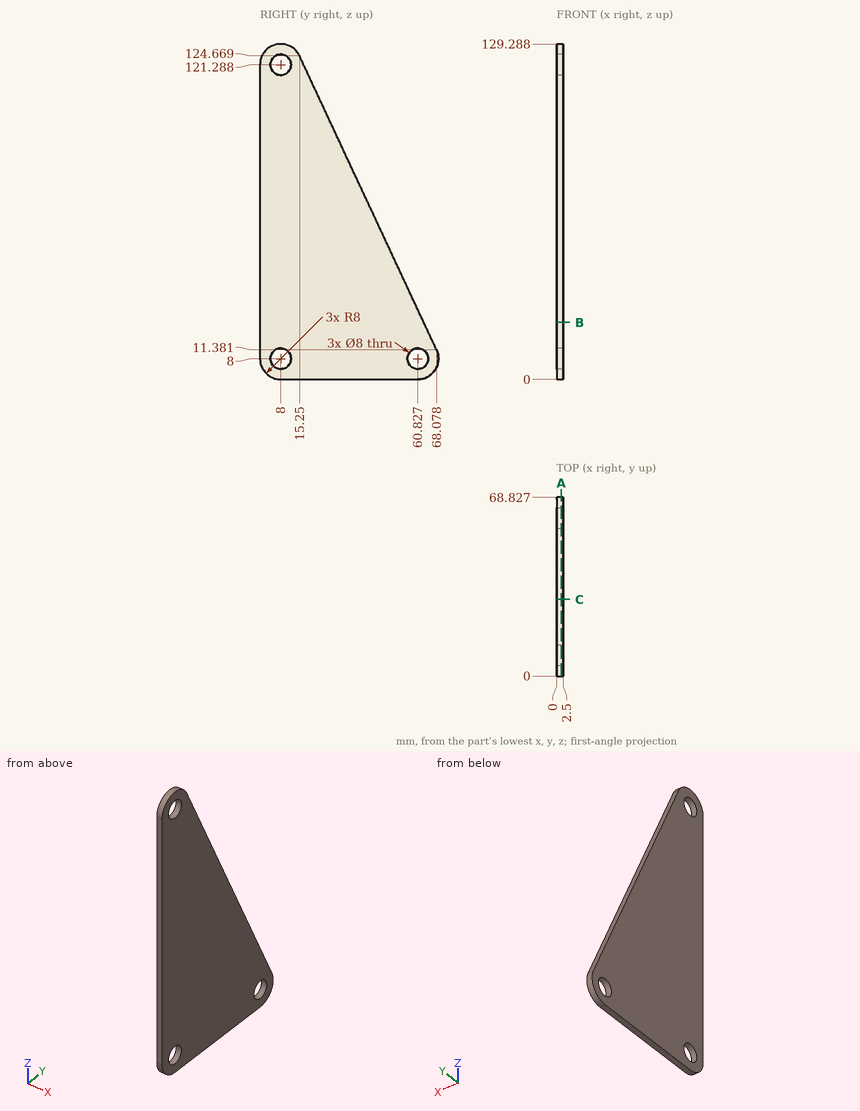
Verification items for this drawing (mm, ordinates from the low corner). Round coordinates to 2 decimals unless told otherwise and drop trailing zeros. Write each loop counter-clockwise with the first axis right and the second up, starting at its lowest first coordinate (ties: lowest second). Pieces come first, ordered by that corner, then holes. Notation, with made-up numbers: (76, -12.5) - (103, -12.5) arc R13 cw to (103, -7.5) - close; hole circle Ø10 at (44, 74). An arc over 180 degrees is marked (long way). Answer as a JSON object with one key per item and string values. Group by question number.
Q1. Go/stop test with a flat-tipped pin: pin 1 Ø1 at (x, z) = (0.5, 104) entering from +Y. Record where the tip stops, or that it passes through.
Q2. Section check C-C, the plane y = 29.5. Enter the section's corners in (x, z).
Q3. Section check B-B, the plane z = 22. Enter the section's corners in (x, y) (1 decimal).
Q4. Thickness scan on line 1 (Y direction, x = 0.85, z = 8); line 2 (Y direction, x = 0.9, z = 121); line 3 (Y direction, x = 0.7, z = 106) (1 decimal). Record the ranges inside material, lowest first.
Q5. Section check A-A, the plane x = 1.9. Enter the section's corners in (y, z).
Found:
{
 "1": {"pin 1": "stops at y = 25.12"},
 "2": {"outline": "(0, 0) - (2.5, 0) - (2.5, 94.11) - (0, 94.11) - close"},
 "3": {"outline": "(0, 0) - (2.5, 0) - (2.5, 63.1) - (0, 63.1) - close"},
 "4": {"line 1": "y = 0 to 4, 12 to 56.83, 64.83 to 68.83", "line 2": "y = 0 to 4.01, 11.99 to 16.96", "line 3": "y = 0 to 24"},
 "5": {"outline": "(0, 8) arc R8 ccw to (8, 0) - (60.83, 0) arc R8 ccw to (68.08, 11.38) - (15.25, 124.67) arc R8 ccw to (0, 121.29) - close; hole circle Ø8 at (8, 8); hole circle Ø8 at (8, 121.29); hole circle Ø8 at (60.83, 8)"}
}
